from build123d import *

# Parameters (mm, degrees)
SKETCH_1_R          = 5
EXTRUDE_1_DEPTH     = 5
SKETCH_2_R          = 4
CUT_EXTRUDE_1_DEPTH = 2.5
SKETCH_3_W          = 32
SKETCH_3_H          = 10
EXTRUDE_2_DEPTH     = 5
CUT_EXTRUDE_2_DEPTH = 20
SKETCH_5_W          = 12
SKETCH_5_H          = 10
CUT_EXTRUDE_3_DEPTH = 5


with BuildPart() as part:
    # 草图1 → 凸台-拉伸1 (new body)
    with BuildSketch(Plane.XY):
        Circle(SKETCH_1_R)
        with BuildLine():
            Line((-40, -5), (0, -5))
            ThreePointArc((0, -5), (-4.095760221, 2.867882182), (4.698463104, 1.710100717))
            Line((4.698463104, 1.710100717), (-3.778366994, 25))
            Line((-3.778366994, 25), (-40, 25))
            Line((-40, 25), (-40, -5))
        make_face()
    extrude(amount=EXTRUDE_1_DEPTH)

    # 草图2 → 切除-拉伸1 (cut)
    with BuildSketch(Plane.XY.offset(5)):
        Circle(SKETCH_2_R)
    extrude(amount=-CUT_EXTRUDE_1_DEPTH, mode=Mode.SUBTRACT)

    # 草图3 → 凸台-拉伸2 (add)
    with BuildSketch(Plane.XY.offset(5)):
        with Locations((-24, 0)):
            Rectangle(SKETCH_3_W, SKETCH_3_H)
    extrude(amount=EXTRUDE_2_DEPTH)

    # 草图4 → 切除-拉伸2 (cut)
    with BuildSketch(Plane(origin=(-8, 0, 0), x_dir=(0, 0, -1), z_dir=(1, 0, 0))):
        Polygon((-10, 4.5), (-5.5, 0), (-10, -4.5), align=None)
    extrude(amount=-CUT_EXTRUDE_2_DEPTH, mode=Mode.SUBTRACT)

    # 草图5 → 切除-拉伸3 (cut)
    with BuildSketch(Plane.XY.offset(10)):
        with Locations((-34, 0)):
            Rectangle(SKETCH_5_W, SKETCH_5_H)
    extrude(amount=-CUT_EXTRUDE_3_DEPTH, mode=Mode.SUBTRACT)


solid = part.part
Verification items for the finished model (mm, model axes). A direction names the side the tool comes from. Round coordinates to 2 decimals unless told otherwise and drop trailing zeros. Write each loop counter-clockwise with the first axis right and the second up, starting at its lowest first coordinate (ties: lowest second). Pieces come first, ordered by that corner, then holes.
(1) Mould release check, pull along X, two halves, no side actions. Record for faces 1 (the flat face through (0, 0, 2.5)), 2 (the cylindrical face through (-0.867, -3.905, 3.768)), 3 (the flat face through (0.52, 13.19, 2.46)), 4 (the flat face through (-22, 25, 2)): pulls with the +X half, pulls with the -X half, needs draft (parallel to the pull), parting line crosses it, or undercut.
Returned:
face 1: undercut
face 2: undercut
face 3: pulls with the +X half
face 4: needs draft
(2) Section check B-B (x = -22). Enter the section's corners in (y, z), plus the area to 3 significant figures.
Returned:
outline: (-5, 0) - (25, 0) - (25, 5) - (5, 5) - (5, 10) - (4.5, 10) - (0, 5.5) - (-4.5, 10) - (-5, 10) - close
area: 180 mm2
(3) Section check C-C (y = 3). Enter the section's corners in (x, z), plus the area to 3 significant figures.
Returned:
outline: (-40, 0) - (4.23, 0) - (4.23, 5) - (2.65, 5) - (2.65, 2.5) - (-2.65, 2.5) - (-2.65, 5) - (-8, 5) - (-8, 8.5) - (-28, 8.5) - (-28, 5) - (-40, 5) - close
area: 278 mm2
(4) Depth check by flat-ended pin: pin 1 Ø2.5 at (y, z) = (0, 7) entering from -X; pin 2 Ø9 at (x, y) = (0, 0) entering from -Z; pin 3 Ø15 at (x, y) = (-15.5, 16.5) entering from +Z; pin 4 Ø1.5 at (y, z) = (-1.5, 7) entering from +X. Enter the tip coordinate at first touch or a pass-through.
Returned:
pin 1: stops at x = -28
pin 2: stops at z = 0
pin 3: stops at z = 5
pin 4: stops at x = -8
(5) Section check A-A (z = 3.25). Enter the section's corners in (x, y).
Returned:
outline: (-40, -5) - (0, -5) arc R5 ccw to (4.7, 1.71) - (-3.78, 25) - (-40, 25) - close; hole circle Ø8 at (0, 0)
(6) Access from +Z, -Z, +X, -X, +Y, -Y to the whole of each face (thin tool, end or side, straight path). Record for faces 5 (the flat face through (-18, 5, 7)), 6 (the flat face through (-28, -1, 6)), 7 (the flat face through (-17.9, -2.2, 7.7)), 8 (the flat face through (-8, -1, 6)), 9 (the flat face through (-20, -5, 4)).
Returned:
face 5: +Z, +X, -X, +Y
face 6: +Z, -X, +Y, -Y
face 7: +Z, +X, -X
face 8: +Z, +X, +Y, -Y
face 9: +Z, -Z, +X, -X, -Y
(7) Section check D-D (y = 6). Enter the section's corners in (x, z), plus the area to 3 significant figures.
Returned:
outline: (-40, 0) - (3.14, 0) - (3.14, 5) - (-40, 5) - close
area: 216 mm2
(8) Material ranges on line 1 (Z direction, x = -17, y = 19); line 2 (Y direction, x = -22.5, z = 7.5); line 3 (Y direction, x = -21.5, z = 6), recorded low to high.
Returned:
line 1: z = 0 to 5
line 2: y = -5 to -2, 2 to 5
line 3: y = -5 to -0.5, 0.5 to 5
